The listing builds one solid part. Answer for the finished solid, in the listing's coordinates (mm). Face numbers are marked on the shaded views. Round coordinates to 2 decimals unless told otherwise and drop trailing zeros. Write each loop counter-clockwise with the first axis right and the second up, starting at its lowest first coordinate (ties: lowest second). Pieces come first, ordered by that corner, then holes. Notation, with made-up numbers: M 66.25,-23.75 L 91.25,-23.75 A32 ccw 91.25,2.25 Z; hole C 45.25,8.25 d5. An arc over 180 degrees is marked long. Write each question's results on one line, items separated by ' | '.
from build123d import *

# Parameters (mm, degrees)
SKIZZE1_W                                           = 65
SKIZZE1_H                                           = 50
AUFSATZ_LINEAR_AUSTRAGEN1_DEPTH                     = 3
VERRUNDUNG1_R                                       = 2
SKIZZE10_R                                          = 4
AUFSATZ_LINEAR_AUSTRAGEN4_DEPTH                     = 2.5
STIRNSENKUNG_F_R_M3_SENKSCHRAUBE_KOPF_B_D           = 4.5
STIRNSENKUNG_F_R_M3_SENKSCHRAUBE_KOPF_B_CBORE_D     = 4.9
STIRNSENKUNG_F_R_M3_SENKSCHRAUBE_KOPF_B_CBORE_DEPTH = 0.3
SKIZZE8_W                                           = 3.5
SKIZZE8_H                                           = 7
AUFSATZ_LINEAR_AUSTRAGEN3_DEPTH                     = 13
STIRNSENKUNG_F_R_M3_SENKSCHRAUBE_KO_2_D             = 2.8
STIRNSENKUNG_F_R_M3_SENKSCHRAUBE_KO_2_CBORE_D       = 6
STIRNSENKUNG_F_R_M3_SENKSCHRAUBE_KO_2_CBORE_DEPTH   = 6
SKIZZE7_W                                           = 1.2
SKIZZE7_H                                           = 3.5
SCHNITT_LINEAR_AUSTRAGEN1_DEPTH                     = 4
VERRUNDUNG2_R                                       = 1.5
VERRUNDUNG5_R                                       = 2.5
VERRUNDUNG6_R                                       = 2.5


with BuildPart() as part:
    # Skizze1 → Aufsatz-Linear austragen1 (new body)
    with BuildSketch(Plane(origin=(0, 0, 0), x_dir=(1, 0, 0), z_dir=(0, 1, 0))):
        with Locations((0, 25)):
            Rectangle(SKIZZE1_W, SKIZZE1_H)
    extrude(amount=AUFSATZ_LINEAR_AUSTRAGEN1_DEPTH)

    # Verrundung1
    verrundung1_edges = [part.edges().sort_by_distance(p)[0] for p in [
        (-32.5, 1.5, -50),
        (32.5, 1.5, -50),
        (32.5, 1.5, 0),
        (-32.5, 1.5, 0),
    ]]
    fillet(verrundung1_edges, radius=VERRUNDUNG1_R)

    # Skizze10 → Aufsatz-Linear austragen4 (add)
    with BuildSketch(Plane(origin=(0, 3, 0), x_dir=(1, 0, 0), z_dir=(0, 1, 0))):
        with Locations((-22.5, 44)):
            Circle(SKIZZE10_R)
        with Locations((-22.5, 19)):
            Circle(SKIZZE10_R)
        with Locations((22.5, 44)):
            Circle(SKIZZE10_R)
        with Locations((22.5, 19)):
            Circle(SKIZZE10_R)
    extrude(amount=AUFSATZ_LINEAR_AUSTRAGEN4_DEPTH)

    # Stirnsenkung f_r M3 Senkschraube _Kopf B (through all)
    with Locations(Plane.XZ):
        with Locations((-22.5, -19), (22.5, -44), (-22.5, -44), (22.5, -19)):
            CounterBoreHole(STIRNSENKUNG_F_R_M3_SENKSCHRAUBE_KOPF_B_D / 2, STIRNSENKUNG_F_R_M3_SENKSCHRAUBE_KOPF_B_CBORE_D / 2, STIRNSENKUNG_F_R_M3_SENKSCHRAUBE_KOPF_B_CBORE_DEPTH)

    # Skizze8 → Aufsatz-Linear austragen3 (add, symmetric)
    with BuildSketch(Plane(origin=(0, 0, 0), x_dir=(0, 0, -1), z_dir=(1, 0, 0))):
        with Locations((5.75, 6.5)):
            Rectangle(SKIZZE8_W, SKIZZE8_H)
    extrude(amount=AUFSATZ_LINEAR_AUSTRAGEN3_DEPTH, both=True)

    # Stirnsenkung f_r M3 Senkschraube _Ko 2 (through all)
    with Locations(Plane(origin=(0, -5, 1.917691722), x_dir=(-1, 0, 0), z_dir=(0, -1, 0))):
        with Locations((9, 7.667691722), (-9, 7.667691722)):
            CounterBoreHole(STIRNSENKUNG_F_R_M3_SENKSCHRAUBE_KO_2_D / 2, STIRNSENKUNG_F_R_M3_SENKSCHRAUBE_KO_2_CBORE_D / 2, STIRNSENKUNG_F_R_M3_SENKSCHRAUBE_KO_2_CBORE_DEPTH)

    # Skizze7 → Schnitt-Linear austragen1 (cut)
    with BuildSketch(Plane(origin=(0, 10, 0), x_dir=(1, 0, 0), z_dir=(0, 1, 0))):
        with Locations((0, 5.75)):
            Rectangle(SKIZZE7_W, SKIZZE7_H)
        with Locations((-5.35, 5.75)):
            Rectangle(SKIZZE7_W, SKIZZE7_H)
        with Locations((5.35, 5.75)):
            Rectangle(SKIZZE7_W, SKIZZE7_H)
    extrude(amount=-SCHNITT_LINEAR_AUSTRAGEN1_DEPTH, mode=Mode.SUBTRACT)

    # Verrundung2
    verrundung2_edges = [part.edges().sort_by_distance(p)[0] for p in [
        (-26.5, 3, -44),
        (-26.5, 3, -19),
        (18.5, 3, -44),
        (18.5, 3, -19),
    ]]
    fillet(verrundung2_edges, radius=VERRUNDUNG2_R)

    # Verrundung5
    verrundung5_edges = [part.edges().sort_by_distance(p)[0] for p in [
        (-13, 3, -5.75),
        (0, 3, -4),
        (13, 3, -5.75),
    ]]
    fillet(verrundung5_edges, radius=VERRUNDUNG5_R)

    # Verrundung6
    verrundung6_edges = [part.edges().sort_by_distance(p)[0] for p in [
        (0, 3, -7.5),
    ]]
    fillet(verrundung6_edges, radius=VERRUNDUNG6_R)


solid = part.part
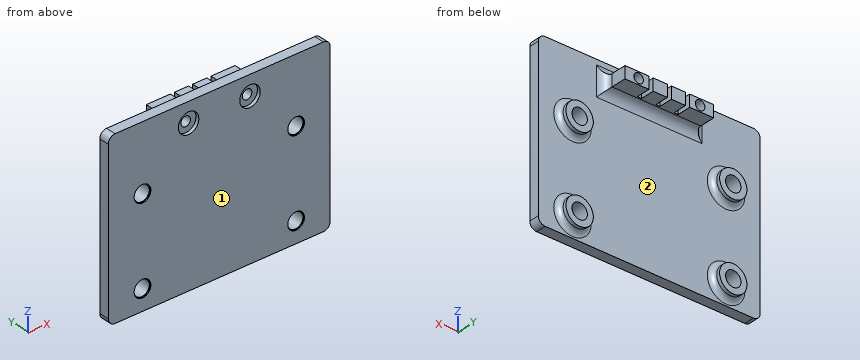
1) Section D-D (y = 1.75) is taken. Determine the outline of the cut face in (x, z).
Return value:
outline: M -32.5,-48 A2 ccw -30.5,-50 L 30.5,-50 A2 ccw 32.5,-48 L 32.5,-2 A2 ccw 30.5,0 L -30.5,0 A2 ccw -32.5,-2 Z; hole C -22.5,-44 d4.5; hole C -22.5,-19 d4.5; hole C -9,-5.75 d2.8; hole C 9,-5.75 d2.8; hole C 22.5,-44 d4.5; hole C 22.5,-19 d4.5
2) Each of these flat-tipped pins is pushed along its axis until it touches: pin 1 (1.8 mm diameter, centred on x = 7.5, z = -6, fed in from -Y); pin 2 (4 mm diameter, centred on x = 22.5, z = -44, fed in from -Y); pin 3 (2.5 mm diameter, centred on x = 23.5, z = -18.5, fed in from -Y); pin 4 (4 mm diameter, centred on y = 6.5, z = -5.5, fed in from -X). Where does it stop, or does it pass through?
Return value:
pin 1: y = 1 | pin 2: through | pin 3: y = 0.3 | pin 4: x = -13.21
3) Section B-B (z = -44) is taken. State how many separate pieces and enclosed holes the cut face has, then the cut area to 3 significant figures.
Return value:
separate pieces: 3 | enclosed holes: 0 | area: 187 mm²
4) Find the intervals of material crossed by line 1 (X direction, y = 7.5, z = -5.75); line 2 (Z direction, x = 22.5, y = 0.1); line 3 (Z direction, x = 9, y = 0.5), in increasing order.
Return value:
line 1: -13 to -10.4, -7.6 to -5.95, -4.75 to -0.6, 0.6 to 4.75, 5.95 to 7.6, 10.4 to 13 | line 2: -50 to -46.45, -41.55 to -21.45, -16.55 to 0 | line 3: -50 to -8.75, -2.75 to 0
5) The mould has two halves that part along X. Classify the marked faces 1 and 2: +X half, -X half, draft (parallel to the pull), parting line (faces both ways), or undercut.
Return value:
face 1: draft | face 2: undercut
6) Section A-A (y = 8.75) is taken. Determine the outline of the cut face in (x, z), then the cut area to 3 significant figures.
Return value:
outline: M -13,-7.5 L -5.95,-7.5 L -5.95,-4 L -13,-4 Z; M -4.75,-7.5 L -0.6,-7.5 L -0.6,-4 L -4.75,-4 Z; M 0.6,-7.5 L 4.75,-7.5 L 4.75,-4 L 0.6,-4 Z; M 5.95,-7.5 L 13,-7.5 L 13,-4 L 5.95,-4 Z; hole C -9,-5.75 d2.8; hole C 9,-5.75 d2.8 | area: 66.1 mm²
